Job drawing, mm, ordinate dimensions from the low corner. One solid piece. A direction names the side the tool comes from. Coordinates: 2 decimals unless noted, no trailing zeros. Loops run counter-clockwise (first coordinate to the right, second up) from the corner with the lowest first, then second, coordinate; pieces in that order, holes last. Notation, with made-up numbers: (52, -9.5) -> (62, -9.5) arc R23 cw to (62, 29.5) -> close; hole circle Ø6 at (78.5, 27). An arc over 180 degrees is marked (long way). Use one line per item in the form item = value. Start each with the question number.
(1) 3-axis set-ups, long thin cutter, end or side, ignore diameter. For the marked faces 4, 5, 6, 7 and 8: which of +Z, -Z, +X, -X, +Y, -Y reach the whole face in a straight line?
(2) Band-saw the part on A-A on y = 17. Give the cut face in (x, z), then the cut area to 3 significant figures.
(3) Mould opens along X. For the marked faces 1, 2 and 3 say: +X half, -X half, draft (parallel to the pull), parting line (faces both ways), or undercut.
(4) Band-saw the part on D-D on z = 19. Give the cut face in (x, y).
(5) Band-saw the part on C-C on y = 4.5. Give the cut face in (x, z).
(6) Band-saw the part on B-B on z = 29. Give the cut face in (x, y), then the cut area to 3 significant figures.
(7) Pin check, flat tips, straight feed: P1, Ø12, axis at x = 40.5, y = 6, coming from the +Z side; P2, Ø4.5, axis at x = 68.5, y = 24.5, coming from the +Z side; P3, Ø15, axis at x = 68.5, z = 30, coming from the +Y side. Stop position of each tip, or through.
(8) Drill centre lines: L1, parallel to X at y = 22.25, z = 44; L2, parallel to X at y = 11.25, z = 28.5; L3, parallel to Z at x = 88.5, y = 22. Where is each one in solid material? Low to high. Write a range as [from, to].
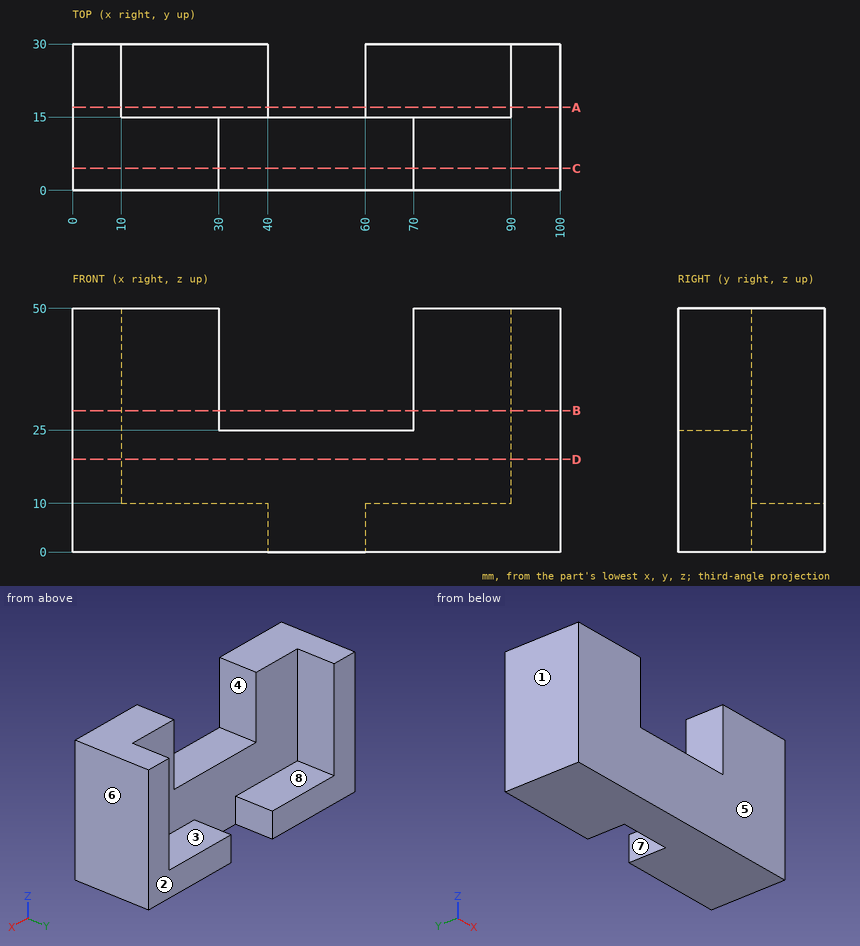
A:
q1.face_4 = +Z, +Y, -Y
q1.face_5 = +Z, -Z, +X, -X, -Y
q1.face_6 = +Z, -Z, +X, +Y, -Y
q1.face_7 = +Z, -Z, +Y
q1.face_8 = +Z, +Y
q2.outline = (0, 0) -> (40, 0) -> (40, 10) -> (10, 10) -> (10, 50) -> (0, 50) -> close; (60, 0) -> (100, 0) -> (100, 50) -> (90, 50) -> (90, 10) -> (60, 10) -> close
q2.area = 1,600 mm²
q3.face_1 = -X half
q3.face_2 = draft
q3.face_3 = undercut
q4.outline = (0, 0) -> (100, 0) -> (100, 30) -> (90, 30) -> (90, 15) -> (10, 15) -> (10, 30) -> (0, 30) -> close
q5.outline = (0, 0) -> (100, 0) -> (100, 50) -> (70, 50) -> (70, 25) -> (30, 25) -> (30, 50) -> (0, 50) -> close
q6.outline = (0, 0) -> (30, 0) -> (30, 15) -> (10, 15) -> (10, 30) -> (0, 30) -> close; (70, 0) -> (100, 0) -> (100, 30) -> (90, 30) -> (90, 15) -> (70, 15) -> close
q6.area = 1,200 mm²
q7.P1 = 25
q7.P2 = 10
q7.P3 = 15
q8.L1 = [0, 10], [90, 100]
q8.L2 = [0, 30], [70, 100]
q8.L3 = [0, 10]
